Part print with two shaded views. Sizes in mm from the minimum x, y, z corner. Give positions to 0.01 mm unless a question says otherwise; leave off trailing zeros. Order: outer loops, then holes, each group sorted by start corner. A loop starts at its lowest first (then second) coordinate and runs counter-clockwise, first axis right, second up.
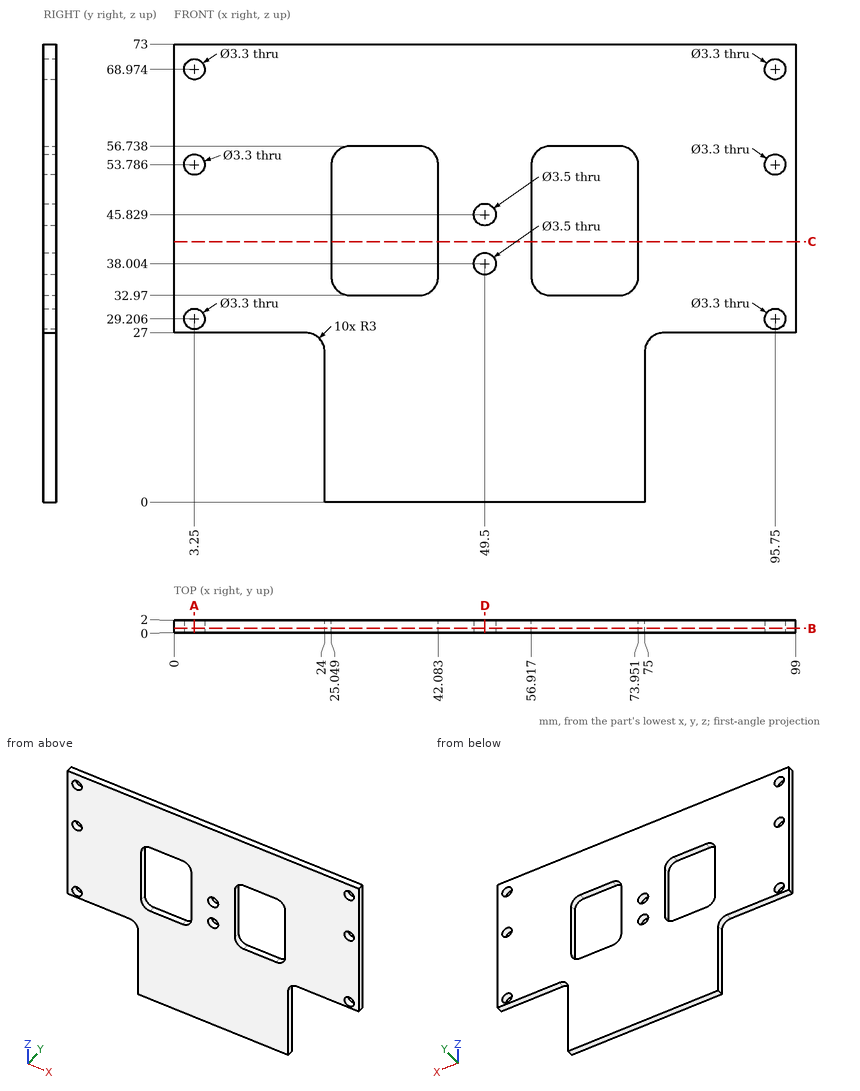
1. Saw through at B-B on y = 0.7. State how many separate pieces and enclosed holes the cut face has, plus the area to 3 significant figures.
2. Saw through at C-C on z = 41.5. Give the cut face in (x, y), plus the area to 3 significant figures.
3. Pin check, flat tips, straight feed: P1, Ø2, axis at x = 95.75, z = 53.79, coming from the +Y side; P2, Ø1, axis at y = 1, z = 24, coming from the -X side; P3, Ø0.6, axis at y = 1.5, z = 14, coming from the +X side. Stop position of each tip, or through.
4. Saw through at D-D on x = 49.5. Give the cut face in (y, z) (1 decimal), plus the area to 3 significant figures.
5. Wall check: line 1 (X direction, y = 1.05, z = 38); line 2 (X direction, y = 1.65, z = 40); line 3 (Z direction, x = 95.75, y = 0.8) (1 decimal). Give the ranges that are in metal, low to high.
6. Saw through at A-A on x = 3.25. Give the cut face in (y, z) (1 decimal).
Reported:
1. separate pieces: 1
1. enclosed holes: 10
1. area: 5,070 mm2
2. outline: (0, 0) - (25.05, 0) - (25.05, 2) - (0, 2) - close; (42.08, 0) - (56.92, 0) - (56.92, 2) - (42.08, 2) - close; (73.95, 0) - (99, 0) - (99, 2) - (73.95, 2) - close
2. area: 130 mm2
3. P1: passes through
3. P2: stops at x = 23.96
3. P3: stops at x = 75
4. outline: (0, 0) - (2, 0) - (2, 36.3) - (0, 36.3) - close; (0, 39.8) - (2, 39.8) - (2, 44.1) - (0, 44.1) - close; (0, 47.6) - (2, 47.6) - (2, 73) - (0, 73) - close
4. area: 132 mm2
5. line 1: x = 0 to 25.05, 42.08 to 47.75, 51.25 to 56.92, 73.95 to 99
5. line 2: x = 0 to 25.05, 42.08 to 56.92, 73.95 to 99
5. line 3: z = 27 to 27.6, 30.9 to 52.1, 55.4 to 67.3, 70.6 to 73
6. outline: (0, 27) - (2, 27) - (2, 27.6) - (0, 27.6) - close; (0, 30.9) - (2, 30.9) - (2, 52.1) - (0, 52.1) - close; (0, 55.4) - (2, 55.4) - (2, 67.3) - (0, 67.3) - close; (0, 70.6) - (2, 70.6) - (2, 73) - (0, 73) - close
